Here's how the part is built. I have some questions about the finished solid (model axes, mm). Give positions to 0.01 mm unless a question says otherwise; leave off trailing zeros. Order: outer loops, then holes, each group sorted by start corner. A loop starts at its lowest first (then second) coordinate and runs counter-clockwise, first axis right, second up. Notation, with made-up numbers: (11.5, 52) -> (67.5, 52) arc R8 ccw to (67.5, 56) -> close; hole circle Ø8 at (6, -10). An arc over 180 degrees is marked (long way). Write each question's results on one line, items separated by ' | '. Start each with the question number.
Q1. Imagine slicing it at C-C, the plane x = 309. Please give me the cut outline in (y, z), then the cut area to 3 significant figures.
Q2. I need wall thicknesses on line 1 along Z through (x, y) = (-61, -9.25); line 2 along X through (y, z) = (-3, 114.5); line 3 along Z through (x, y) = (-156.5, -9.5). Which ranges of each line are inside material? Lowest first, please. Write a range as [from, to].
Q3. I'm going to push flat-ended pins straight in: pin 1 (4.5 mm diameter, centred on x = 246.5, y = -5, fed in from -Z); pin 2 (4.5 mm diameter, centred on y = -8, z = 24, fed in from +X); pin 3 (2 mm diameter, centred on y = -11, z = 93, fed in from +X). Where does each tip first touch, or does it pass through?
Q4. Imagine slicing it at A-A, the plane z = -24. State how many separate pieces and enclosed holes the cut face has, then the cut area to 3 significant figures.
```python
from build123d import *

# Parameters (mm, degrees)
F1_DEPTH = 15


# Not quite as in the source:
# - ends of sketch curves that miss each other by under 0.0002 mm in the source are joined


with BuildPart() as f1:
    # F0 (on Front) → F1 (new body)
    with BuildSketch(Plane.XZ):
        with BuildLine():
            Line((152.4, -104.775), (152.4, -114.3))
            ThreePointArc((152.4, -114.3), (156.1197438789, -123.2802561211), (165.1, -127))
            Line((165.1, -127), (215.9, -127))
            ThreePointArc((215.9, -127), (224.8802561211, -123.2802561211), (228.6, -114.3))
            Line((228.6, -114.3), (228.6, -104.775))
            ThreePointArc((228.6, -104.775), (229.5299359697, -102.5299359697), (231.775, -101.6))
            Line((231.775, -101.6), (265.179556, -101.6))
            ThreePointArc((265.179556, -101.6), (272.1974896575, -99.4848291048), (276.8777652022, -93.8438751462))
            Line((276.8777652022, -93.8438751462), (357.711629, 97.4253068))
            ThreePointArc((357.711629, 97.4253068), (365.0341452454, 100.3972108736), (368.0060482736, 93.0746921546))
            Line((368.0060482736, 93.0746921546), (361.9191644, 78.6719534))
            ThreePointArc((361.9191644, 78.6719534), (362.4758586154, 72.6910380462), (367.7682764, 69.85))
            Line((367.7682764, 69.85), (376.592338, 69.85))
            ThreePointArc((376.592338, 69.85), (380.1013055832, 70.9075859478), (382.4414433059, 73.7280640946))
            Line((382.4414433059, 73.7280640946), (397.4984938, 109.3561186))
            ThreePointArc((397.4984938, 109.3561186), (396.3851270368, 121.3179295371), (385.8002952, 127))
            Line((385.8002952, 127), (-351.0556098, 127))
            ThreePointArc((-351.0556098, 127), (-361.6404416368, 121.3179295371), (-362.7538151531, 109.356115746))
            Line((-362.7538151531, 109.356115746), (-359.6258238, 101.9546856))
            ThreePointArc((-359.6258238, 101.9546856), (-362.1924804362, 95.6306809293), (-368.5164757001, 98.1973326577))
            Line((-368.5164757001, 98.1973326577), (-377.411107, 119.2438814))
            ThreePointArc((-377.411107, 119.2438814), (-380.76124871, 123.8707639235), (-385.8003211895, 126.5613398156))
            ThreePointArc((-385.8003211895, 126.5613398156), (-387.4548258, 126.780671), (-389.1093307052, 126.5613409078))
            ThreePointArc((-389.1093307052, 126.5613409078), (-397.2156200075, 119.8660524106), (-397.4985259531, 109.356115746))
            Line((-397.4985259531, 109.356115746), (-311.6224908, -93.8438814))
            ThreePointArc((-311.6224908, -93.8438814), (-306.9422004575, -99.4848291048), (-299.9242668, -101.6))
            Line((-299.9242668, -101.6), (-231.775, -101.6))
            ThreePointArc((-231.775, -101.6), (-229.5299359697, -102.5299359697), (-228.6, -104.775))
            Line((-228.6, -104.775), (-228.6, -114.3))
            ThreePointArc((-228.6, -114.3), (-224.8802561211, -123.2802561211), (-215.9, -127))
            Line((-215.9, -127), (-165.1, -127))
            ThreePointArc((-165.1, -127), (-156.1197438789, -123.2802561211), (-152.4, -114.3))
            Line((-152.4, -114.3), (-152.4, -104.775))
            ThreePointArc((-152.4, -104.775), (-151.4700640303, -102.5299359697), (-149.225, -101.6))
            Line((-149.225, -101.6), (-41.275, -101.6))
            ThreePointArc((-41.275, -101.6), (-39.0299359697, -102.5299359697), (-38.1, -104.775))
            Line((-38.1, -104.775), (-38.1, -114.3))
            ThreePointArc((-38.1, -114.3), (-34.3802561211, -123.2802561211), (-25.4, -127))
            Line((-25.4, -127), (25.4, -127))
            ThreePointArc((25.4, -127), (34.3802561211, -123.2802561211), (38.1, -114.3))
            Line((38.1, -114.3), (38.1, -104.775))
            ThreePointArc((38.1, -104.775), (39.0299359697, -102.5299359697), (41.275, -101.6))
            Line((41.275, -101.6), (149.225, -101.6))
            ThreePointArc((149.225, -101.6), (151.4700640303, -102.5299359697), (152.4, -104.775))
        make_face()
        with BuildLine():
            ThreePointArc((-215.9, -53.848), (-218.727005348, -60.672994652), (-225.552, -63.5))
            Line((-225.552, -63.5), (-231.648, -63.5))
            ThreePointArc((-231.648, -63.5), (-238.472994652, -60.672994652), (-241.3, -53.848))
            Line((-241.3, -53.848), (-241.3, 79.248))
            ThreePointArc((-241.3, 79.248), (-238.472994652, 86.072994652), (-231.648, 88.9))
            Line((-231.648, 88.9), (-225.552, 88.9))
            ThreePointArc((-225.552, 88.9), (-218.727005348, 86.072994652), (-215.9, 79.248))
            Line((-215.9, 79.248), (-215.9, -53.848))
        make_face(mode=Mode.SUBTRACT)
        with BuildLine():
            ThreePointArc((-139.7, -53.848), (-142.527005348, -60.672994652), (-149.352, -63.5))
            Line((-149.352, -63.5), (-155.448, -63.5))
            ThreePointArc((-155.448, -63.5), (-162.272994652, -60.672994652), (-165.1, -53.848))
            Line((-165.1, -53.848), (-165.1, 79.248))
            ThreePointArc((-165.1, 79.248), (-162.272994652, 86.072994652), (-155.448, 88.9))
            Line((-155.448, 88.9), (-149.352, 88.9))
            ThreePointArc((-149.352, 88.9), (-142.527005348, 86.072994652), (-139.7, 79.248))
            Line((-139.7, 79.248), (-139.7, -53.848))
        make_face(mode=Mode.SUBTRACT)
        with BuildLine():
            ThreePointArc((-63.5, -53.848), (-66.327005348, -60.672994652), (-73.152, -63.5))
            Line((-73.152, -63.5), (-79.248, -63.5))
            ThreePointArc((-79.248, -63.5), (-86.072994652, -60.672994652), (-88.9, -53.848))
            Line((-88.9, -53.848), (-88.9, 79.248))
            ThreePointArc((-88.9, 79.248), (-86.072994652, 86.072994652), (-79.248, 88.9))
            Line((-79.248, 88.9), (-73.152, 88.9))
            ThreePointArc((-73.152, 88.9), (-66.327005348, 86.072994652), (-63.5, 79.248))
            Line((-63.5, 79.248), (-63.5, -53.848))
        make_face(mode=Mode.SUBTRACT)
        with BuildLine():
            ThreePointArc((12.7, -53.848), (9.872994652, -60.672994652), (3.048, -63.5))
            Line((3.048, -63.5), (-3.048, -63.5))
            ThreePointArc((-3.048, -63.5), (-9.872994652, -60.672994652), (-12.7, -53.848))
            Line((-12.7, -53.848), (-12.7, 79.248))
            ThreePointArc((-12.7, 79.248), (-9.872994652, 86.072994652), (-3.048, 88.9))
            Line((-3.048, 88.9), (3.048, 88.9))
            ThreePointArc((3.048, 88.9), (9.872994652, 86.072994652), (12.7, 79.248))
            Line((12.7, 79.248), (12.7, -53.848))
        make_face(mode=Mode.SUBTRACT)
        with BuildLine():
            ThreePointArc((88.9, -53.848), (86.072994652, -60.672994652), (79.248, -63.5))
            Line((79.248, -63.5), (73.152, -63.5))
            ThreePointArc((73.152, -63.5), (66.327005348, -60.672994652), (63.5, -53.848))
            Line((63.5, -53.848), (63.5, 79.248))
            ThreePointArc((63.5, 79.248), (66.327005348, 86.072994652), (73.152, 88.9))
            Line((73.152, 88.9), (79.248, 88.9))
            ThreePointArc((79.248, 88.9), (86.072994652, 86.072994652), (88.9, 79.248))
            Line((88.9, 79.248), (88.9, -53.848))
        make_face(mode=Mode.SUBTRACT)
        with BuildLine():
            ThreePointArc((165.1, -53.848), (162.272994652, -60.672994652), (155.448, -63.5))
            Line((155.448, -63.5), (149.352, -63.5))
            ThreePointArc((149.352, -63.5), (142.527005348, -60.672994652), (139.7, -53.848))
            Line((139.7, -53.848), (139.7, 79.248))
            ThreePointArc((139.7, 79.248), (142.527005348, 86.072994652), (149.352, 88.9))
            Line((149.352, 88.9), (155.448, 88.9))
            ThreePointArc((155.448, 88.9), (162.272994652, 86.072994652), (165.1, 79.248))
            Line((165.1, 79.248), (165.1, -53.848))
        make_face(mode=Mode.SUBTRACT)
        with BuildLine():
            ThreePointArc((241.3, -53.848), (238.472994652, -60.672994652), (231.648, -63.5))
            Line((231.648, -63.5), (225.552, -63.5))
            ThreePointArc((225.552, -63.5), (218.727005348, -60.672994652), (215.9, -53.848))
            Line((215.9, -53.848), (215.9, 79.248))
            ThreePointArc((215.9, 79.248), (218.727005348, 86.072994652), (225.552, 88.9))
            Line((225.552, 88.9), (231.648, 88.9))
            ThreePointArc((231.648, 88.9), (238.472994652, 86.072994652), (241.3, 79.248))
            Line((241.3, 79.248), (241.3, -53.848))
        make_face(mode=Mode.SUBTRACT)
    extrude(amount=F1_DEPTH)


solid = f1.part
```
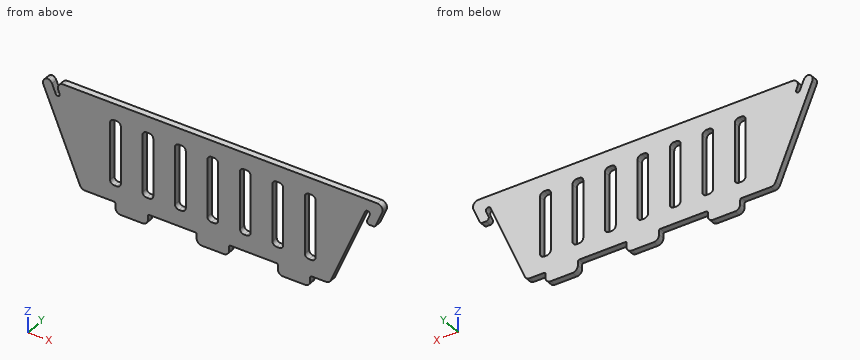
Geometry check:
1) outline: (-15, -17.84) -> (0, -17.84) -> (0, 127) -> (-15, 127) -> close | area: 2,170 mm²
2) line 1: [-101.6, 127] | line 2: [-398.5, -375.41], [-363.75, 398.5] | line 3: [-123.65, -63.44], [88.84, 127]
3) pin 1: z = -101.6 | pin 2: x = 327.63 | pin 3: x = 391.01
4) separate pieces: 8 | enclosed holes: 0 | area: 7,050 mm²
